Part model, mm, in its own coordinate system. Coordinates: 2 decimals unless noted, no trailing zeros. Order: outer loops, then holes, each group sorted by start corner. A loop starts at its lowest first (then second) coordinate and runs counter-clockwise, first axis right, second up.
1) Cut at B-B (y = 19.5). List the corners of the cut face in (x, z), and give its area (3 significant figures).
2) Cut at C-C (x = 35). List the corners of the cut face in (y, z).
3) Cut at A-A (x = 68). List the corners of the cut face in (y, z).
4) Cut at D-D (z = 1.45). Give the number of separate pieces and of enclosed holes in the cut face, and give its area (3 significant figures).
5) Pin check, flat tips, straight feed: pin 1 Ø0.9 at (x, z) = (-15, 2) entering from -Y; pin 2 Ø2 at (x, y) = (3.5, 20.5) entering from +Z; pin 3 Ø0.9 at (x, z) = (33.5, 1) entering from +Y; pin 4 Ø0.9 at (y, z) = (12, 1.5) entering from +X. Stop position of each tip, or through.
6) Wall check: L1, parallel to Y at x = 0, z = 0.8; L2, parallel to Y at x = 2, z = 1.3; L3, parallel to X at y = 24, z = 1.85. Give the ranges that are in metal, low to high.
```python
from build123d import *

# Parameters (mm, degrees)
F0_R     = 4.2
F1_DEPTH = 3
F3_DEPTH = 3
F4_R     = 5
F5_R     = 2


with BuildPart() as f1:
    # F0 (on Top) → F1 (new body)
    with BuildSketch(Plane.XY):
        with BuildLine():
            ThreePointArc((6.545227, 3), (7.034402, 1.535312), (7.2, 0))
            Line((7.2, 0), (30, 0))
            Line((30, 0), (38, 0))
            Line((38, 0), (60.8, 0))
            ThreePointArc((60.8, 0), (60.965598, 1.535312), (61.454773, 3))
            Line((61.454773, 3), (41.167184, 3))
            ThreePointArc((41.167184, 3), (68, 27), (94.832816, 3))
            Line((94.832816, 3), (74.545227, 3))
            ThreePointArc((74.545227, 3), (75.034402, 1.535312), (75.2, 0))
            Line((75.2, 0), (98, 0))
            ThreePointArc((98, 0), (75.764571, 28.977775), (42.019238, 15))
            Line((42.019238, 15), (25.980762, 15))
            ThreePointArc((25.980762, 15), (-7.764571, 28.977775), (-30, 0))
            Line((-30, 0), (-7.2, 0))
            ThreePointArc((-7.2, 0), (-7.034402, 1.535312), (-6.545227, 3))
            Line((-6.545227, 3), (-26.832816, 3))
            ThreePointArc((-26.832816, 3), (0, 27), (26.832816, 3))
            Line((26.832816, 3), (6.545227, 3))
        make_face()
        with BuildLine():
            Line((38.150377, 3), (29.849623, 3))
            ThreePointArc((29.849623, 3), (29.023516, 7.591807), (27.495454, 12))
            Line((27.495454, 12), (40.504546, 12))
            ThreePointArc((40.504546, 12), (38.976484, 7.591807), (38.150377, 3))
        make_face(mode=Mode.SUBTRACT)
        with BuildLine():
            ThreePointArc((-7.2, 0), (0, -7.2), (7.2, 0))
            ThreePointArc((7.2, 0), (7.034402, 1.535312), (6.545227, 3))
            ThreePointArc((6.545227, 3), (0, 7.2), (-6.545227, 3))
            ThreePointArc((-6.545227, 3), (-7.034402, 1.535312), (-7.2, 0))
        make_face()
        Circle(F0_R, mode=Mode.SUBTRACT)
        with BuildLine():
            ThreePointArc((61.454773, 3), (60.965598, 1.535312), (60.8, 0))
            ThreePointArc((60.8, 0), (68, -7.2), (75.2, 0))
            ThreePointArc((75.2, 0), (75.034402, 1.535312), (74.545227, 3))
            ThreePointArc((74.545227, 3), (68, 7.2), (61.454773, 3))
        make_face()
        with Locations((68, 0)):
            Circle(F0_R, mode=Mode.SUBTRACT)
    extrude(amount=F1_DEPTH)

    # F2 (on face) → F3 (join, through all)
    with BuildSketch(Plane.XY.offset(3)):
        with BuildLine():
            Line((1.5, 7.042017), (1.5, 26.958301))
            ThreePointArc((1.5, 26.958301), (0.75029, 26.989573), (0, 27))
            Line((0, 27), (0, 7.2))
            ThreePointArc((0, 7.2), (0.754148, 7.160395), (1.5, 7.042017))
        make_face()
        with BuildLine():
            Line((0, 7.2), (0, 27))
            ThreePointArc((0, 27), (-0.75029, 26.989573), (-1.5, 26.958301))
            Line((-1.5, 26.958301), (-1.5, 7.042017))
            ThreePointArc((-1.5, 7.042017), (-0.754148, 7.160395), (0, 7.2))
        make_face()
        with BuildLine():
            Line((68, 7.2), (68, 27))
            ThreePointArc((68, 27), (67.24971, 26.989573), (66.5, 26.958301))
            Line((66.5, 26.958301), (66.5, 7.042017))
            ThreePointArc((66.5, 7.042017), (67.245852, 7.160395), (68, 7.2))
        make_face()
        with BuildLine():
            Line((69.5, 7.042017), (69.5, 26.958301))
            ThreePointArc((69.5, 26.958301), (68.75029, 26.989573), (68, 27))
            Line((68, 27), (68, 7.2))
            ThreePointArc((68, 7.2), (68.754148, 7.160395), (69.5, 7.042017))
        make_face()
    extrude(amount=-F3_DEPTH)

    # F4
    f4_edges = [f1.edges().sort_by_distance(p)[0] for p in [
        (-26.832816, 3, 1.5),
        (26.832816, 3, 1.5),
        (94.832816, 3, 1.5),
        (41.167184, 3, 1.5),
        (-7.2, 0, 1.5),
        (7.2, 0, 1.5),
        (60.8, 0, 1.5),
        (75.2, 0, 1.5),
        (74.545227, 3, 1.5),
        (61.454773, 3, 1.5),
        (-6.545227, 3, 1.5),
        (6.545227, 3, 1.5),
        (25.980762, 15, 1.5),
        (42.019238, 15, 1.5),
        (98, 0, 1.5),
        (-30, 0, 1.5),
        (-1.5, 7.042017, 1.5),
        (1.5, 7.042017, 1.5),
        (1.5, 26.958301, 1.5),
        (-1.5, 26.958301, 1.5),
        (69.5, 26.958301, 1.5),
        (66.5, 26.958301, 1.5),
    ]]
    fillet(f4_edges, radius=F4_R)

    # F5
    f5_edges = [f1.edges().sort_by_distance(p)[0] for p in [
        (27.495454, 12, 1.5),
        (40.504546, 12, 1.5),
        (29.849623, 3, 1.5),
        (38.150377, 3, 1.5),
    ]]
    fillet(f5_edges, radius=F5_R)


solid = f1.part
```
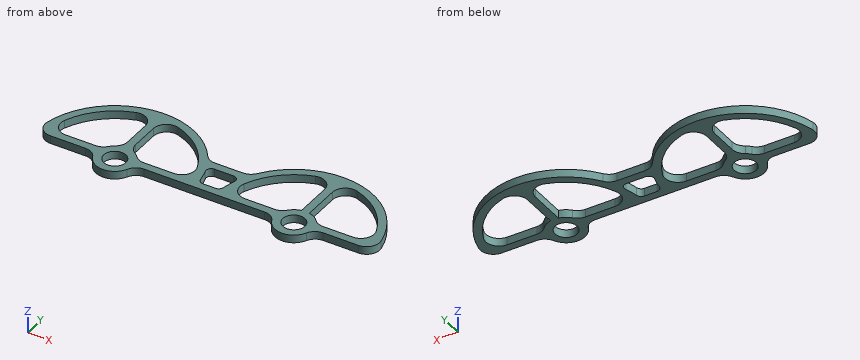
Geometry check:
1. outline: (-22.8, 0) - (-18.67, 0) - (-18.67, 3) - (-22.8, 3) - close; (-1.5, 0) - (1.5, 0) - (1.5, 3) - (-1.5, 3) - close; (18.67, 0) - (22.8, 0) - (22.8, 3) - (18.67, 3) - close; (45.2, 0) - (49.33, 0) - (49.33, 3) - (45.2, 3) - close; (66.5, 0) - (69.5, 0) - (69.5, 3) - (66.5, 3) - close; (86.67, 0) - (90.8, 0) - (90.8, 3) - (86.67, 3) - close
1. area: 67.5 mm2
2. outline: (0, 0) - (3, 0) - (3, 3) - (0, 3) - close; (12, 0) - (15, 0) - (15, 3) - (12, 3) - close
3. outline: (-7.2, 0) - (-4.2, 0) - (-4.2, 3) - (-7.2, 3) - close; (4.2, 0) - (30, 0) - (30, 3) - (4.2, 3) - close
4. separate pieces: 1
4. enclosed holes: 7
4. area: 1,260 mm2
5. pin 1: stops at y = 0
5. pin 2: passes through
5. pin 3: stops at y = 15
5. pin 4: stops at x = 95.69
6. L1: y = -7.2 to -4.2, 4.2 to 30
6. L2: y = -6.92 to -3.69, 3.69 to 8.14, 23.2 to 29.93
6. L3: x = -18 to -12.37, -2.49 to 2.49, 12.37 to 18, 50 to 55.63, 65.51 to 70.49, 80.37 to 86
